Build history of the part. All positions in model axes, mm. Face numbers are marked on the shaded views. Give positions to 0.01 mm unless a question says otherwise; leave off trailing zeros. Write each loop counter-clockwise with the first axis right and the second up, starting at its lowest first coordinate (ties: lowest second). Pieces come first, ordered by that corner, then holes. Notation, with made-up numbers: (-5, -13) -> (41, -13) arc R21 ccw to (41, 3) -> close; hole circle Ø4 at (60, 80). An arc over 180 degrees is marked (long way). Put each result on its own line as item: value.
from build123d import *

# Parameters (mm, degrees)
F1_DEPTH    = 21
F2_R        = 10.5
F3_DEPTH    = 25
F4_T1_DEPTH = 30.3938312155
F5_R        = 14
F6_DEPTH    = 25


# Not quite as in the source:
# - a fillet or chamfer that OpenCascade refuses, or shapes differently, is made with other operations: its cross-section is extruded or revolved along the edge and cut away or added


with BuildPart() as f1:
    # F0 (on Right) → F1 (new body)
    with BuildSketch(Plane.YZ):
        Polygon((-134.9917307664, 26.4616465569), (-134.9917307664, -3.5383534431), (-39.9917307664, -43.5383534431), (190.0082692336, -43.5383534431), (190.0082692336, 26.4616465569), align=None)
    extrude(amount=F1_DEPTH)

    # F2 (on face) → F3 (cut)
    with BuildSketch(Plane.YZ.offset(21)):
        with Locations((163.0082692336, 22.4616465569)):
            Circle(F2_R)
        with Locations((109.0082692336, 22.4616465569)):
            Circle(F2_R)
        with Locations((55.0082692336, 22.4616465569)):
            Circle(F2_R)
        with Locations((1.0082692336, 22.4616465569)):
            Circle(F2_R)
        with Locations((-52.9917307664, 22.4616465569)):
            Circle(F2_R)
        with Locations((-106.9917307664, 22.4616465569)):
            Circle(F2_R)
    extrude(amount=-F3_DEPTH, mode=Mode.SUBTRACT)

    # F4: chamfer of 2 on 10 edges, made by hand

    # F4_s2 → F4_t1 (cut)
    with BuildSketch(Plane.YZ.offset(-4.6969156077)):
        with BuildLine():
            Line((-64.5776976071, 26.5242502898), (-63.1732755163, 24.7590076766))
            Line((-63.1732755163, 24.7590076766), (-63.1342989368, 24.7500173343))
            ThreePointArc((-63.1342989368, 24.7500173343), (-62.963845112, 25.6189453198), (-62.6629908996, 26.4464084616))
            Line((-62.6629908996, 26.4464084616), (-62.6999746859, 26.5016465569))
            ThreePointArc((-62.6999746859, 26.5016465569), (-63.6388361465, 26.5016465569), (-64.5776976071, 26.5642502898))
            Line((-64.5776976071, 26.5642502898), (-64.5776976071, 26.5242502898))
        make_face()
        with BuildLine():
            Line((-42.8101860166, 24.7590076766), (-41.4057639258, 26.5242502898))
            Line((-41.4057639258, 26.5242502898), (-41.4057639258, 26.5642502898))
            ThreePointArc((-41.4057639258, 26.5642502898), (-42.3446253864, 26.5016465569), (-43.283486847, 26.5016465569))
            Line((-43.283486847, 26.5016465569), (-43.3204706333, 26.4464084616))
            ThreePointArc((-43.3204706333, 26.4464084616), (-43.0196164209, 25.6189453198), (-42.8491625961, 24.7500173343))
            Line((-42.8491625961, 24.7500173343), (-42.8101860166, 24.7590076766))
        make_face()
        with BuildLine():
            Line((-10.5776976071, 26.5242502898), (-9.1732755163, 24.7590076766))
            Line((-9.1732755163, 24.7590076766), (-9.1342989368, 24.7500173343))
            ThreePointArc((-9.1342989368, 24.7500173343), (-8.963845112, 25.6189453198), (-8.6629908996, 26.4464084616))
            Line((-8.6629908996, 26.4464084616), (-8.6999746859, 26.5016465569))
            ThreePointArc((-8.6999746859, 26.5016465569), (-9.6388361465, 26.5016465569), (-10.5776976071, 26.5642502898))
            Line((-10.5776976071, 26.5642502898), (-10.5776976071, 26.5242502898))
        make_face()
        with BuildLine():
            Line((11.1898139834, 24.7590076766), (12.5942360742, 26.5242502898))
            Line((12.5942360742, 26.5242502898), (12.5942360742, 26.5642502898))
            ThreePointArc((12.5942360742, 26.5642502898), (11.6553746136, 26.5016465569), (10.716513153, 26.5016465569))
            Line((10.716513153, 26.5016465569), (10.6795293667, 26.4464084616))
            ThreePointArc((10.6795293667, 26.4464084616), (10.9803835791, 25.6189453198), (11.1508374039, 24.7500173343))
            Line((11.1508374039, 24.7500173343), (11.1898139834, 24.7590076766))
        make_face()
        with BuildLine():
            Line((43.4223023929, 26.5242502898), (44.8267244837, 24.7590076766))
            Line((44.8267244837, 24.7590076766), (44.8657010632, 24.7500173343))
            ThreePointArc((44.8657010632, 24.7500173343), (45.036154888, 25.6189453198), (45.3370091004, 26.4464084616))
            Line((45.3370091004, 26.4464084616), (45.3000253141, 26.5016465569))
            ThreePointArc((45.3000253141, 26.5016465569), (44.3611638535, 26.5016465569), (43.4223023929, 26.5642502898))
            Line((43.4223023929, 26.5642502898), (43.4223023929, 26.5242502898))
        make_face()
        with BuildLine():
            Line((65.1898139834, 24.7590076766), (66.5942360742, 26.5242502898))
            Line((66.5942360742, 26.5242502898), (66.5942360742, 26.5642502898))
            ThreePointArc((66.5942360742, 26.5642502898), (65.6553746136, 26.5016465569), (64.716513153, 26.5016465569))
            Line((64.716513153, 26.5016465569), (64.6795293667, 26.4464084616))
            ThreePointArc((64.6795293667, 26.4464084616), (64.9803835791, 25.6189453198), (65.1508374039, 24.7500173343))
            Line((65.1508374039, 24.7500173343), (65.1898139834, 24.7590076766))
        make_face()
        with BuildLine():
            Line((97.4223023929, 26.5242502898), (98.8267244837, 24.7590076766))
            Line((98.8267244837, 24.7590076766), (98.8657010632, 24.7500173343))
            ThreePointArc((98.8657010632, 24.7500173343), (99.036154888, 25.6189453198), (99.3370091004, 26.4464084616))
            Line((99.3370091004, 26.4464084616), (99.3000253141, 26.5016465569))
            ThreePointArc((99.3000253141, 26.5016465569), (98.3611638535, 26.5016465569), (97.4223023929, 26.5642502898))
            Line((97.4223023929, 26.5642502898), (97.4223023929, 26.5242502898))
        make_face()
        with BuildLine():
            Line((119.1898139834, 24.7590076766), (120.5942360742, 26.5242502898))
            Line((120.5942360742, 26.5242502898), (120.5942360742, 26.5642502898))
            ThreePointArc((120.5942360742, 26.5642502898), (119.6553746136, 26.5016465569), (118.716513153, 26.5016465569))
            Line((118.716513153, 26.5016465569), (118.6795293667, 26.4464084616))
            ThreePointArc((118.6795293667, 26.4464084616), (118.9803835791, 25.6189453198), (119.1508374039, 24.7500173343))
            Line((119.1508374039, 24.7500173343), (119.1898139834, 24.7590076766))
        make_face()
        with BuildLine():
            Line((151.4223023929, 26.5242502898), (152.8267244837, 24.7590076766))
            Line((152.8267244837, 24.7590076766), (152.8657010632, 24.7500173343))
            ThreePointArc((152.8657010632, 24.7500173343), (153.036154888, 25.6189453198), (153.3370091004, 26.4464084616))
            Line((153.3370091004, 26.4464084616), (153.3000253141, 26.5016465569))
            ThreePointArc((153.3000253141, 26.5016465569), (152.3611638535, 26.5016465569), (151.4223023929, 26.5642502898))
            Line((151.4223023929, 26.5642502898), (151.4223023929, 26.5242502898))
        make_face()
        with BuildLine():
            Line((173.1898139834, 24.7590076766), (174.5942360742, 26.5242502898))
            Line((174.5942360742, 26.5242502898), (174.5942360742, 26.5642502898))
            ThreePointArc((174.5942360742, 26.5642502898), (173.6553746136, 26.5016465569), (172.716513153, 26.5016465569))
            Line((172.716513153, 26.5016465569), (172.6795293667, 26.4464084616))
            ThreePointArc((172.6795293667, 26.4464084616), (172.9803835791, 25.6189453198), (173.1508374039, 24.7500173343))
            Line((173.1508374039, 24.7500173343), (173.1898139834, 24.7590076766))
        make_face()
    extrude(amount=F4_T1_DEPTH, mode=Mode.SUBTRACT)

    # F5 (on face) → F6 (cut)
    with BuildSketch(Plane.YZ.offset(21)):
        with Locations((-21.4917307664, -43.5383534431)):
            Circle(F5_R)
    extrude(amount=-F6_DEPTH, mode=Mode.SUBTRACT)


solid = f1.part
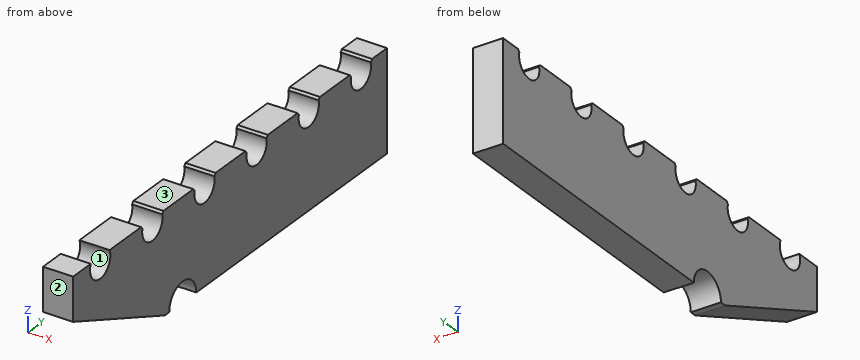
1) Slice it at D-D (z = -20.5). Write the cut outline in (x, y).
Filled sheet:
outline: (0, -94.71) -> (21, -94.71) -> (21, 190.01) -> (0, 190.01) -> close
2) Pull direction Y, two halves, no side cores. Call the marked faces 1, 2 and 3: released by +Y, released by -Y, zero draft, split by the parting line, or undercut.
Filled sheet:
face 1: undercut
face 2: released by -Y
face 3: zero draft
3) Slice it at B-B (z = 17). Write the cut outline in (x, y).
Filled sheet:
outline: (0, -134.99) -> (21, -134.99) -> (21, -115.96) -> (0, -115.96) -> close; (0, -98.02) -> (21, -98.02) -> (21, -61.96) -> (0, -61.96) -> close; (0, -44.02) -> (21, -44.02) -> (21, -7.96) -> (0, -7.96) -> close; (0, 9.98) -> (21, 9.98) -> (21, 46.04) -> (0, 46.04) -> close; (0, 63.98) -> (21, 63.98) -> (21, 100.04) -> (0, 100.04) -> close; (0, 117.98) -> (21, 117.98) -> (21, 154.04) -> (0, 154.04) -> close; (0, 171.98) -> (21, 171.98) -> (21, 190.01) -> (0, 190.01) -> close
4) Pin check, flat tips, straight feed: pin 1 (2 mm diameter, centred on x = 14.5, y = 48, fed in from +Z); pin 2 (12 mm diameter, centred on y = 121, z = 14.5, fed in from -X); pin 3 (5 mm diameter, centred on x = 3, y = -25.5, fed in from -Z); pin 4 (1.5 mm diameter, centred on x = 14.5, y = -76.5, fed in from -Z). Stop position of each tip, or through.
Filled sheet:
pin 1: z = 15.67
pin 2: x = 0
pin 3: z = -31.14
pin 4: z = -28.48
5) Slice it at C-C (y = 50). Write the cut outline in (x, z), plus the area to 3 significant figures.
Filled sheet:
outline: (0, -43.54) -> (21, -43.54) -> (21, 13.23) -> (0, 13.23) -> close
area: 1,190 mm2
6) Wall check: L1, parallel to Y at x = 6, z = -37; L2, parallel to Y at x = 13.25, z = -36; L3, parallel to Z at x = 7, y = 109. Give the ranges that are in metal, low to high.
Filled sheet:
L1: -55.52 to -33.87, -9.11 to 190.01
L2: -57.9 to -33.29, -9.69 to 190.01
L3: -43.54 to 11.96
